CAD build for the part. Positions are in the model's coordinates, mm. Face numbers are marked on the shaded views. A direction names the side the tool comes from. Coordinates: 2 decimals unless noted, no trailing zeros. Loops run counter-clockwise (first coordinate to the right, second up) from the corner with the lowest first, then second, coordinate; pieces in that order, holes last.
1) Pin check, flat tips, straight feed: pin 1 Ø3 at (x, y) = (20, 20.5) entering from +Z; pin 2 Ø3 at (y, z) = (18, 1.5) entering from -X; pin 3 Ø1.5 at (x, z) = (12, 15) entering from +Y; pin 4 Ø5.5 at (y, z) = (18.5, -1.5) entering from +X. Stop position of each tip, or through.
2) Saw through at D-D, the plane y = 4.75. Write the cut outline in (x, z), and give its area (3 significant figures).
3) Saw through at B-B, the plane y = 21. Write the cut outline in (x, z), and give its area (3 significant figures).
4) Two-plate mould, pull along X, no slides. Class the marked faces 1, 2, 3 and 4: +X half, -X half, draft (parallel to the pull), parting line (faces both ways), or undercut.
5) Which spindle directions (+Z, -Z, +X, -X, +Y, -Y) get a long thin tool onto all of the face, cutting with end or side? Do the marked faces 5, 6, 7 and 8. Say none if no direction does.
6) Wall check: line 1 along Y through (x, z) = (6.5, 3.1); line 2 along Y through (x, z) = (6, 3) (3 decimals); line 3 along Z through (x, y) = (12, 6). Give the ranges that are in metal, low to high.
7) Saw through at C-C, the plane z = 15. Write the cut outline in (x, y), and give its area (3 significant figures).
8) Saw through at A-A, the plane x = 18.5. Write the cut outline in (y, z), and give its area (3 significant figures).
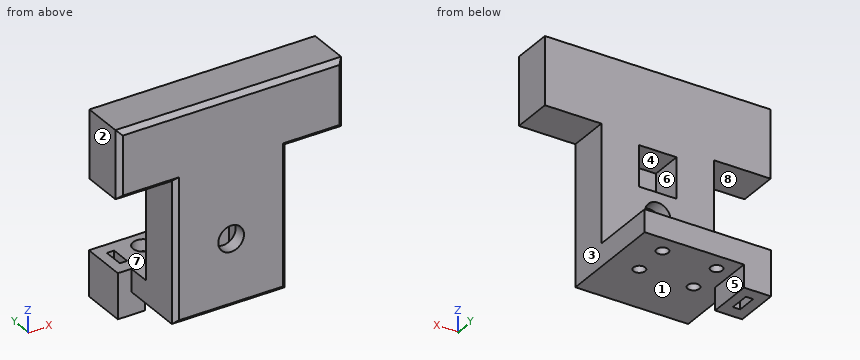
```python
from build123d import *

# Parameters (mm, degrees)
SKETCH1_W                      = 25
SKETCH1_H                      = 25
BOSS_EXTRUDE1_DEPTH            = 5
CBORE_FOR_M2_SHCS1_D           = 2.6
CBORE_FOR_M2_SHCS1_CBORE_D     = 4.6
CBORE_FOR_M2_SHCS1_CBORE_DEPTH = 2.6
SKETCH5_W                      = 25
SKETCH5_H                      = 10
BOSS_EXTRUDE2_DEPTH            = 26
SKETCH6_R                      = 2.85
CUT_EXTRUDE1_DEPTH             = 43.555845662
SKETCH7_W                      = 8.3
SKETCH7_H                      = 4.3
CUT_EXTRUDE2_DEPTH             = 22
SKETCH8_W                      = 8.3
SKETCH8_H                      = 9
CUT_EXTRUDE3_DEPTH             = 2.85
SKETCH7_2_W                    = 8.3
SKETCH7_2_H                    = 4.3
BOSS_EXTRUDE5_DEPTH            = 2
SKETCH9_W                      = 50
SKETCH9_H                      = 10
BOSS_EXTRUDE3_DEPTH            = 20
SKETCH10_W                     = 50
SKETCH10_H                     = 7
CUT_EXTRUDE4_DEPTH             = 66.055745327
SKETCH11_W                     = 5
SKETCH11_H                     = 25
BOSS_EXTRUDE6_DEPTH            = 3
SKETCH12_W                     = 3
SKETCH12_H                     = 15
CUT_EXTRUDE5_DEPTH             = 60.600755029
SKETCH13_W                     = 6
SKETCH13_H                     = 10
BOSS_EXTRUDE7_DEPTH            = 5
SKETCH14_W                     = 1.219
SKETCH14_H                     = 4.08
CUT_EXTRUDE6_DEPTH             = 60.600755029
SKETCH15_W                     = 1.619
SKETCH15_H                     = 4.48
CUT_EXTRUDE7_DEPTH             = 60.600755029
SKETCH16_W                     = 50
SKETCH16_H                     = 10
BOSS_EXTRUDE8_DEPTH            = 2
CHAMFER1_SIZE                  = 1


with BuildPart() as part:
    # Sketch1 → Boss-Extrude1 (new body)
    with BuildSketch(Plane.XY):
        with Locations((12.5, 12.5)):
            Rectangle(SKETCH1_W, SKETCH1_H)
    extrude(amount=BOSS_EXTRUDE1_DEPTH)

    # CBORE for M2 SHCS1 (through all)
    with Locations(Plane.XY.offset(5)):
        with Locations((6.5, 21), (18.5, 21), (18.5, 13), (6.5, 13)):
            CounterBoreHole(CBORE_FOR_M2_SHCS1_D / 2, CBORE_FOR_M2_SHCS1_CBORE_D / 2, CBORE_FOR_M2_SHCS1_CBORE_DEPTH)

    # Sketch5 → Boss-Extrude2 (add)
    with BuildSketch(Plane.XY.offset(5)):
        with Locations((12.5, 5)):
            Rectangle(SKETCH5_W, SKETCH5_H)
    extrude(amount=BOSS_EXTRUDE2_DEPTH)

    # Sketch6 → Cut-Extrude1 (cut, through all)
    with BuildSketch(Plane(origin=(0, 10, 0), x_dir=(1, 0, 0), z_dir=(0, 1, 0))):
        with Locations(Location((12.5, -15, 0), (0, 0, 270))):
            Circle(SKETCH6_R)
    extrude(amount=-CUT_EXTRUDE1_DEPTH, mode=Mode.SUBTRACT)

    # Sketch7 → Cut-Extrude2 (cut)
    with BuildSketch(Plane.XY.offset(31)):
        with Locations((12.5, 5)):
            Rectangle(SKETCH7_W, SKETCH7_H)
    extrude(amount=-CUT_EXTRUDE2_DEPTH, mode=Mode.SUBTRACT)

    # Sketch8 → Cut-Extrude3 (cut)
    with BuildSketch(Plane(origin=(0, 10, 0), x_dir=(1, 0, 0), z_dir=(0, 1, 0))):
        with Locations((12.5, -24.5)):
            Rectangle(SKETCH8_W, SKETCH8_H)
    extrude(amount=-CUT_EXTRUDE3_DEPTH, mode=Mode.SUBTRACT)

    # Sketch7<2> → Boss-Extrude5 (add)
    with BuildSketch(Plane.XY.offset(31)):
        with Locations((12.5, 5)):
            Rectangle(SKETCH7_2_W, SKETCH7_2_H)
    extrude(amount=-BOSS_EXTRUDE5_DEPTH)

    # Sketch9 → Boss-Extrude3 (add)
    with BuildSketch(Plane.XY.offset(31)):
        with Locations((12.5, 5)):
            Rectangle(SKETCH9_W, SKETCH9_H)
    extrude(amount=BOSS_EXTRUDE3_DEPTH)

    # Sketch10 → Cut-Extrude4 (cut, through all)
    with BuildSketch(Plane(origin=(0, 10, 0), x_dir=(1, 0, 0), z_dir=(0, 1, 0))):
        with Locations((12.5, -47.5)):
            Rectangle(SKETCH10_W, SKETCH10_H)
    extrude(amount=-CUT_EXTRUDE4_DEPTH, mode=Mode.SUBTRACT)

    # Sketch11 → Boss-Extrude6 (add)
    with BuildSketch(Plane.ZY):
        with Locations((2.5, 12.5)):
            Rectangle(SKETCH11_W, SKETCH11_H)
    extrude(amount=BOSS_EXTRUDE6_DEPTH)

    # Sketch12 → Cut-Extrude5 (cut, through all)
    with BuildSketch(Plane.XY.offset(5)):
        with Locations((-1.5, 7.5)):
            Rectangle(SKETCH12_W, SKETCH12_H)
    extrude(amount=-CUT_EXTRUDE5_DEPTH, mode=Mode.SUBTRACT)

    # Sketch13 → Boss-Extrude7 (add)
    with BuildSketch(Plane(origin=(0, 0, 0), x_dir=(-1, 0, 0), z_dir=(0, 0, -1))):
        with Locations((0, 20)):
            Rectangle(SKETCH13_W, SKETCH13_H)
    extrude(amount=BOSS_EXTRUDE7_DEPTH)

    # Sketch14 → Cut-Extrude6 (cut, through all)
    with BuildSketch(Plane.XY.offset(5)):
        with Locations((0.0895, 20.12)):
            Rectangle(SKETCH14_W, SKETCH14_H)
    extrude(amount=-CUT_EXTRUDE6_DEPTH, mode=Mode.SUBTRACT)

    # Sketch15 → Cut-Extrude7 (cut, through all)
    with BuildSketch(Plane.XY.offset(5)):
        with Locations((0.0895, 20.12)):
            Rectangle(SKETCH15_W, SKETCH15_H)
    extrude(amount=-CUT_EXTRUDE7_DEPTH, mode=Mode.SUBTRACT)

    # Sketch16 → Boss-Extrude8 (add)
    with BuildSketch(Plane.XY.offset(44)):
        with Locations((12.5, 5)):
            Rectangle(SKETCH16_W, SKETCH16_H)
    extrude(amount=BOSS_EXTRUDE8_DEPTH)

    # Chamfer1
    chamfer1_edges = [part.edges().sort_by_distance(p)[0] for p in [
        (-6.25, 0, 31),
        (31.25, 0, 31),
        (37.5, 0, 38.5),
        (-12.5, 0, 38.5),
        (12.5, 0, 0),
        (12.5, 0, 46),
        (25, 0, 15.5),
        (0, 0, 15.5),
    ]]
    chamfer(chamfer1_edges, length=CHAMFER1_SIZE)


solid = part.part
```
Data:
1. pin 1: stops at z = 5
1. pin 2: stops at x = -3
1. pin 3: passes through
1. pin 4: stops at x = 25
2. outline: (-12.5, 31) - (0, 31) - (0, 0) - (25, 0) - (25, 31) - (37.5, 31) - (37.5, 46) - (-12.5, 46) - close; hole (8.35, 9) - (16.65, 9) - (16.65, 29) - (8.35, 29) - close
2. area: 1,360 mm2
3. outline: (-3, -5) - (-0.72, -5) - (-0.72, 5) - (-3, 5) - close; (0.9, -5) - (3, -5) - (3, 0) - (5.2, 0) - (5.2, 2.4) - (4.2, 2.4) - (4.2, 5) - (0.9, 5) - close; (7.8, 0) - (17.2, 0) - (17.2, 2.4) - (16.2, 2.4) - (16.2, 5) - (8.8, 5) - (8.8, 2.4) - (7.8, 2.4) - close; (19.8, 0) - (25, 0) - (25, 5) - (20.8, 5) - (20.8, 2.4) - (19.8, 2.4) - close
3. area: 117 mm2
4. face 1: draft
4. face 2: -X half
4. face 3: +X half
4. face 4: undercut
5. face 5: -Z, +X, +Y, -Y
5. face 6: none
5. face 7: +Z, +X, -X, +Y
5. face 8: -Z, -X, +Y, -Y
6. line 1: y = 0 to 10.7, 15.3 to 18.7, 23.3 to 25
6. line 2: y = 0 to 10.755, 15.245 to 18.755, 23.245 to 25
6. line 3: z = 0 to 9, 29 to 46
7. outline: (0, 1) - (1, 0) - (9.65, 0) - (9.65, 2.85) - (8.35, 2.85) - (8.35, 7.15) - (9.65, 7.15) - (9.65, 10) - (0, 10) - close; (15.35, 0) - (24, 0) - (25, 1) - (25, 10) - (15.35, 10) - (15.35, 7.15) - (16.65, 7.15) - (16.65, 2.85) - (15.35, 2.85) - close
7. area: 181 mm2
8. outline: (0, 1) - (1, 0) - (11.7, 0) - (11.7, 2.4) - (10.7, 2.4) - (10.7, 5) - (10, 5) - (10, 46) - (1, 46) - (0, 45) - close; (14.3, 0) - (19.7, 0) - (19.7, 2.4) - (18.7, 2.4) - (18.7, 5) - (15.3, 5) - (15.3, 2.4) - (14.3, 2.4) - close; (22.3, 0) - (25, 0) - (25, 5) - (23.3, 5) - (23.3, 2.4) - (22.3, 2.4) - close
8. area: 498 mm2
